Autodesk Inventor part; units mm, degrees
ref_plane "YZ Plane" through (0, 0, 0) normal (1, 0, 0) x (0, 1, 0)
ref_plane "XZ Plane" through (0, 0, 0) normal (0, 1, 0) x (-1, 0, 0)
ref_plane "XY Plane" through (0, 0, 0) normal (0, 0, 1) x (1, 0, 0)
sketch "Sketch1" plane through (0, 0, 0) normal (0, 0, 1) x (1, 0, 0)
  line L0 (11.43, 7.62) -> (0, 7.62)
  arc A0 (0, 7.62) -> (0, -7.62) centre (0, 0) ccw
  line L1 (0, -7.62) -> (11.43, -7.62)
  line L2 (11.43, -7.62) -> (11.43, 7.62)
  dimension "d0" = 15.24
  dimension "d2" = 11.43
extrude "Extrusion1" add sketch "Sketch1" along normal blind 8.89
sketch "Sketch2" plane through (0, 0, 8.89) normal (0, 0, 1) x (1, 0, 0)
  arc A0 (0, 7.62) -> (0, -7.62) centre (0, 0) ccw
  circle A1 centre (0, 0) radius 5.08
  dimension "d5" = 10.16
extrude "Extrusion2" add sketch "Sketch2" along normal blind 10.16
sketch "Sketch3" plane through (0, 0, 0) normal (0, 1, 0) x (-1, 0, 0)
  line L0 (7.62, 8.89) -> (7.62, 0)
  line L1 (7.62, 0) -> (-11.43, 0)
  line L2 (-11.43, 0) -> (-11.43, 8.89)
  line L3 (-11.43, 8.89) -> (-5.08, 8.89)
  line L4 (-5.08, 8.89) -> (-5.08, 19.05)
  line L5 (-5.08, 19.05) -> (5.08, 19.05)
  line L6 (5.08, 19.05) -> (5.08, 8.89)
  line L7 (5.08, 8.89) -> (7.62, 8.89)
  line L8 (0, 19.05) -> (0, 38.1)
  arc A0 (3.175, 37.465) -> (0, 38.1) centre (0, 29.845) ccw
  arc A1 (3.175, 37.465) -> (3.175, 27.432) centre (16.8842, 32.4485) ccw
  line L9 (3.175, 27.432) -> (3.175, 19.05)
  line L10 (3.175, 19.05) -> (0, 19.05)
  line L11 (16.8842, 32.4485) -> (2.286, 32.4485)
  point P0 (0, 0)
  dimension "d10" = 3.175
  dimension "d13" = 8.382
  dimension "d14" = 2.286
  dimension "d15" = 19.05
  dimension "d16" = 0.635
revolve "Revolution1" add sketch "Sketch3" angle 360 about axis through (0, 0, 19.05) along (0, 0, 1) contours L5 L8 A0 A1 L9
sketch "Sketch4" plane through (0, 0, 0) normal (0, 1, 0) x (-1, 0, 0)
  line L0 (7.62, 8.89) -> (7.62, 0)
  line L1 (7.62, 0) -> (-11.43, 0)
  line L2 (-11.43, 0) -> (-11.43, 8.89)
  line L3 (-11.43, 8.89) -> (-5.08, 8.89)
  line L4 (-5.08, 8.89) -> (-5.08, 19.05)
  line L5 (-5.08, 19.05) -> (-3.175, 19.05)
  line L6 (-3.175, 19.05) -> (-3.175, 27.432)
  arc A0 (-3.175, 27.432) -> (-3.175, 37.465) centre (-16.8842, 32.4485) ccw
  arc A1 (3.175, 37.465) -> (0, 38.1) centre (0, 29.845) ccw
  arc A2 (0, 38.1) -> (-3.175, 37.465) centre (0, 29.845) ccw
  arc A3 (3.175, 37.465) -> (3.175, 27.432) centre (16.8842, 32.4485) ccw
  line L7 (3.175, 27.432) -> (3.175, 19.05)
  line L8 (3.175, 19.05) -> (5.08, 19.05)
  line L9 (5.08, 19.05) -> (5.08, 8.89)
  line L10 (5.08, 8.89) -> (7.62, 8.89)
  circle A4 centre (0, 32.4485) radius 1.27
  point P0 (0, 0)
  point P1 (2.286, 32.4485)
  dimension "d18" = 2.54
extrude "Extrusion3" cut sketch "Sketch4" along normal through all both and the other way through all contours A4
sketch "Sketch5" plane through (0, 0, 8.89) normal (0, 0, 1) x (1, 0, 0)
  circle A0 centre (0, 0) radius 5.08
  arc A1 (0, 7.62) -> (0, -7.62) centre (0, 0) ccw
  line L0 (-1.7571, 7.4147) -> (-5.8207, 10.24)
  arc A2 (-5.8207, 10.24) -> (-10.24, 5.8207) centre (-7.6332, 7.6332) ccw
  line L1 (-10.24, 5.8207) -> (-7.4147, 1.7571)
  circle A3 centre (-7.6332, 7.6332) radius 1.125
  circle A4 centre (0, 0) radius 10.795
  line L2 (0, 0) -> (-7.6332, 7.6332)
  line L3 (11.43, 7.62) -> (0, 7.62)
  dimension "d23" = 2.25
  dimension "d25" = 3.175
  dimension "d26" = 8.001
  dimension "d27" = 5.715
  dimension "d31" = 135
extrude "Extrusion4" add sketch "Sketch5" against normal blind 2.159 contours A1 L1 A4 A3 L2 | L2 A3 A4 L0 A1 | A4 A3 L1 A2 L0
fillet "Fillet1" radius 4.4 1 edges at (11.43, 0, 0)
sketch "Sketch6" plane through (0, -7.62, 8.89) normal (0, -1, 0) x (1, 0, 0)
  arc A0 (7.03, -8.89) -> (11.43, -4.49) centre (7.03, -4.49) ccw
  circle A1 centre (7.03, -4.49) radius 3.81
  dimension "d33" = 7.62
extrude "Extrusion5" add sketch "Sketch6" along normal blind 11.43
sketch "Sketch7" plane through (7.03, -19.05, 4.4) normal (0, -1, 0) x (1, 0, 0)
  circle A0 centre (0, 0) radius 3.81
  line L0 (-10.541, 2.54) -> (10.541, 2.54)
  line L1 (10.541, 2.54) -> (10.541, -2.54)
  line L2 (10.541, -2.54) -> (-10.541, -2.54)
  line L3 (-10.541, -2.54) -> (-10.541, 2.54)
  point P0 (-7.03, -4.4)
  point P1 (0, 2.54)
  point P2 (10.541, 0)
  dimension "d37" = 21.082
  dimension "d40" = 5.08
extrude "Extrusion6" add sketch "Sketch7" along normal blind 15.24 contours A0 L2 L0 | A0 L0 L1 L2 | A0 L2 L3 L0
sketch "Sketch8" plane through (-3.511, -19.05, 6.94) normal (0, 0, 1) x (1, 0, 0)
  line L0 (0, 0) -> (7.7012, 0)
  line L1 (0, 0) -> (0, -15.24)
  line L2 (21.082, -15.24) -> (0, -15.24)
  line L3 (21.082, 0) -> (21.082, -15.24)
  line L4 (13.3808, 0) -> (21.082, 0)
  line L5 (7.7012, 0) -> (13.3808, 0)
  line L6 (6.1817, 0) -> (0, -3.7039)
  line L7 (14.9003, 0) -> (21.082, -3.7039)
  arc A0 (0, -12.9438) -> (21.082, -12.9438) centre (10.541, 10.1034) ccw
  point P0 (3.511, 19.05)
extrude "Extrusion7" cut sketch "Sketch8" against normal through all contours L0 L6 L1 | A0 L2 L1 | A0 L3 L2 | L4 L3 L7
properties part number "tuning peg"
Input: part model. Units: mm. Frame: model coordinates. A direction names the side the tool comes from. Round coordinates to 2 decimals unless told otherwise and drop trailing zeros. Loops run counter-clockwise (first coordinate to the right, second up) from the corner with the lowest first, then second, coordinate; pieces in that order, holes last. Notation, with made-up numbers: M 19.25,85.5 L 62.25,85.5 A16 cw 62.25,115.5 Z; hole C 29,58.5 d9. An arc over 180 degrees is marked long. Answer as CSV lines item,"result". Start each with the question number.
(1) Line query: line 1 (Z direction, x = 0, y = 0.3); line 2 (Z direction, x = 9.25, y = -26); line 3 (Z direction, x = -5.75, y = 7). Output: solid intervals per line, ascending. Write a range as [from, to].
(2) First-contact query: pin 1 (2 mm diameter, centred on x = -7.63, y = 7.63, fed in from -Z); pin 2 (4.5 mm diameter, centred on x = 6.5, z = 3, fed in from -Y); pin 3 (4 mm diameter, centred on y = 2, z = 26.5, fed in from +X) (3 decimals); pin 4 (4.5 mm diameter, centred on x = 3, y = -27, fed in from +Z). Flat tips, straight axial feed; report the tip coordinate or a pass-through.
(3) Section D-D, the plane y = -17.5. Output: boundary loops of the cut face in (x, z).
(4) Reachability of faces 1 (the cylindrical face through (0.69, -3.1, 23.18)), 2 (the flat face through (3, -7.62, 4)), 3 (the flat face through (-3.511, -27, 4)) from +Z, -Z, +X, -X, +Y, -Y: full face, straight path, thin tool, end or side. Return the list, or none.
(5) Draft query along Y for faces 4 (the flat face through (-0.38, -20.88, 4.44)), 5 (the flat face through (7, -27, 1.86)), 6 (the cylindrical face through (-9.834, 9.922, 7.826)), 7 (the flat face through (3, -19.05, 4)). Return one class per face: released by +Y, released by -Y, zero draft, split by the parting line, or undercut.
(6) Section B-B, the plane x = 8. Output: boundary loops of the cut face in (y, z).
(7) Section C-C, the plane z = 12. Output: boundary loops of the cut face in (x, y).
Values found:
1,line 1,"z = [0, 31.18], [33.72, 38.09]"
1,line 2,"z = [1.86, 6.94]"
1,line 3,"z = [6.73, 8.89]"
2,pin 1,"passes through"
2,pin 2,"stops at y = -34.29"
2,pin 3,"stops at x = 3.175"
2,pin 4,"stops at z = 6.94"
3,outline,"C 7.03,4.4 d7.62"
4,face 1,"+Z"
4,face 2,"none"
4,face 3,"+Z, -Z, -X, -Y"
5,face 4,"undercut"
5,face 5,"zero draft"
5,face 6,"split by the parting line"
5,face 7,"undercut"
6,outline,"M -34.27,1.86 L -19.05,1.86 L -19.05,0.72 L -7.62,0.72 L -7.62,0.11 L 7.62,0.11 L 7.62,8.89 L -7.62,8.89 L -7.62,8.08 L -19.05,8.08 L -19.05,6.94 L -34.27,6.94 Z"
7,outline,"C 0,0 d10.16"
